Model file for the job. Use its own axes, mm. Round coordinates to 2 decimals unless told otherwise and drop trailing zeros. Order: outer loops, then holes, each group sorted by start corner. A loop starts at its lowest first (then second) coordinate and runs counter-clockwise, first axis right, second up. Notation, with made-up numbers: (-0.75, -7.5) - (49.25, -7.5) arc R23 cw to (49.25, 25.5) - close; hole circle Ø10 at (22, 0). An arc over 180 degrees is marked (long way). Put each result on its own line as item: value. Start each with the question number.
Item 1: Probe probe 1 along X at (y, z) = (50, -0.7); probe 2 along Y at (x, z) = (127.5, -0.2); probe 3 along X at (y, z) = (-41, -0.3). List the from-to ranges inside material, lowest first.
Item 2: Saw through at B-B on x = -143.5. List the corners of the cut face in (y, z).
Item 3: Saw through at A-A on z = -0.7. State how many separate pieces and enclosed holes the cut face has, plus the area to 3 significant figures.
Item 4: Saw through at C-C on y = -54. List the corners of the cut face in (x, z).
```python
from build123d import *

# Parameters (mm, degrees)
BASE_FLANGE1_DEPTH                 = 1
F_4_2_START                        = -1
F_4_2_4_2_DIAMETER_HOLE1_OUTLINE_R = 2.1
F_4_2_4_2_DIAMETER_HOLE1_DEPTH     = 1


# Read off the part's stored shape, not the designer's step: Ø4.2 (4.2) Diameter Hole1
# Sheet-metal steps are written as plain solids
with BuildPart() as part:
    # Sketch1 → Base-Flange1 (new body)
    with BuildSketch(Plane.XY):
        with BuildLine():
            Line((-120.688391142, 62.855752194), (-211.490666647, -45.358185855))
            ThreePointArc((-211.490666647, -45.358185855), (-213.594616806, -61.339273926), (-200, -70))
            Line((-200, -70), (150, -70))
            ThreePointArc((150, -70), (164.142135624, -64.142135624), (170, -50))
            Line((170, -50), (170, -13.032012463))
            ThreePointArc((170, -13.032012463), (171.206147584, -6.191609597), (174.679111138, -0.176260269))
            Line((174.679111138, -0.176260269), (195.320888862, 24.423652492))
            ThreePointArc((195.320888862, 24.423652492), (198.793852416, 30.439001819), (200, 37.279404685))
            Line((200, 37.279404685), (200, 60))
            ThreePointArc((200, 60), (197.071067812, 67.071067812), (190, 70))
            Line((190, 70), (-105.36750228, 70))
            ThreePointArc((-105.36750228, 70), (-113.819867515, 68.126155741), (-120.688391142, 62.855752194))
        make_face()
    extrude(amount=-BASE_FLANGE1_DEPTH)

    # Ø4.2 (4.2) Diameter Hole1 outline → Ø4.2 (4.2) Diameter Hole1 (cut)
    with BuildSketch(Plane.XY.offset(F_4_2_START)):
        with Locations((107.976556815, -41.6)):
            Circle(F_4_2_4_2_DIAMETER_HOLE1_OUTLINE_R)
        with Locations((69.42162602, -41.6)):
            Circle(F_4_2_4_2_DIAMETER_HOLE1_OUTLINE_R)
        with Locations((-133.690845807, -42.192339034)):
            Circle(F_4_2_4_2_DIAMETER_HOLE1_OUTLINE_R)
        with Locations((-172.245776602, -42.192339034)):
            Circle(F_4_2_4_2_DIAMETER_HOLE1_OUTLINE_R)
        with Locations((-74.698274088, 49.596767959)):
            Circle(F_4_2_4_2_DIAMETER_HOLE1_OUTLINE_R)
        with Locations((126.46596136, -9.64433534)):
            Circle(F_4_2_4_2_DIAMETER_HOLE1_OUTLINE_R)
        with Locations((-97.693405311, 49.596767959)):
            Circle(F_4_2_4_2_DIAMETER_HOLE1_OUTLINE_R)
        with Locations((126.46596136, 28.910595455)):
            Circle(F_4_2_4_2_DIAMETER_HOLE1_OUTLINE_R)
    extrude(amount=F_4_2_4_2_DIAMETER_HOLE1_DEPTH, mode=Mode.SUBTRACT)


solid = part.part
```
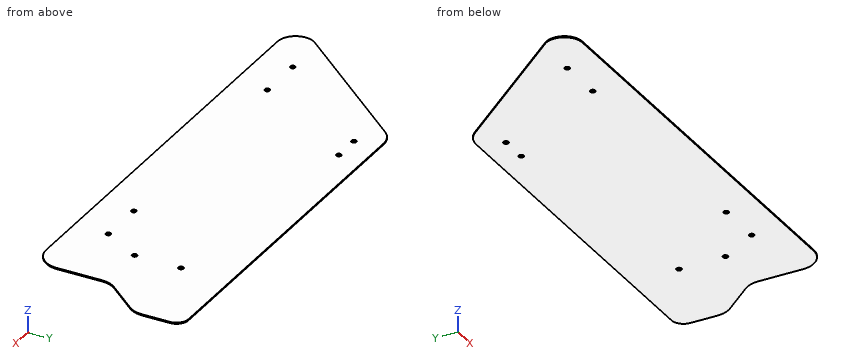
Results found:
1. probe 1: x = -131.48 to -99.75, -95.63 to -76.76, -72.64 to 200
1. probe 2: y = -70 to -11.47, -7.82 to 27.08, 30.74 to 70
1. probe 3: x = -207.83 to -173.97, -170.52 to -135.42, -131.96 to 67.41, 71.43 to 105.96, 109.99 to 170
2. outline: (-70, -1) - (35.67, -1) - (35.67, 0) - (-70, 0) - close
3. separate pieces: 1
3. enclosed holes: 8
3. area: 49,400 mm²
4. outline: (-214.97, -1) - (169.6, -1) - (169.6, 0) - (-214.97, 0) - close
